Design review of the part built by this model. Coordinates are the model's own, in mm. A direction names the side the tool comes from. Give positions to 0.01 mm unless a question says otherwise; leave off trailing zeros. Loops run counter-clockwise (first coordinate to the right, second up) from the corner with the lowest first, then second, coordinate; pieces in that order, holes last. Notation, with made-up numbers: M -35.5,1 L -0.5,1 A20 ccw -0.5,25 Z; hole C -23.5,28.5 d8. An arc over 180 degrees is marked long. Use one line per item in the form item = value. Start each with the question number.
Autodesk Inventor part; units mm, degrees
ref_plane "YZ Plane" through (0, 0, 0) normal (1, 0, 0) x (0, 1, 0)
ref_plane "XZ Plane" through (0, 0, 0) normal (0, 1, 0) x (-1, 0, 0)
ref_plane "XY Plane" through (0, 0, 0) normal (0, 0, 1) x (1, 0, 0)
sketch "Sketch1" plane through (0, 0, 0) normal (0, 1, 0) x (-1, 0, 0)
  line L0 (25, 25) -> (-25, 25)
  line L1 (-25, 25) -> (-25, -25)
  line L2 (-25, -25) -> (25, -25)
  line L3 (25, -25) -> (25, 25)
  point P0 (0, 0)
  dimension "d0" = 50
  dimension "d1" = 50
  dimension "d2" = 25
  dimension "d3" = 25
extrude "Extrusion1" add sketch "Sketch1" along normal blind 7.5
sketch "Sketch2" plane through (0, 7.5, 0) normal (0, 1, 0) x (1, 0, 0)
  line L0 (-25, 25) -> (-25, -25)
  line L1 (25, -25) -> (25, 25)
  line L2 (-25, -25) -> (25, -25)
  line L3 (25, -25) -> (25, -17.5)
  line L4 (25, -17.5) -> (-25, -17.5)
  line L5 (-25, -17.5) -> (-25, -25)
  line L6 (-25, 25) -> (25, 25)
  line L7 (25, 25) -> (25, 17.5)
  line L8 (25, 17.5) -> (-25, 17.5)
  line L9 (-25, 17.5) -> (-25, 25)
  point P0 (0, 0)
  point P1 (-25, -17.5)
  point P2 (-25, 17.5)
  dimension "d6" = 7.5
  dimension "d7" = 7.5
  dimension "d8" = 25
extrude "Extrusion2" add sketch "Sketch2" along normal blind 120 contours L6 L1 L8 L0 | L4 L1 L2 L0
sketch "Sketch3" plane through (-25, 0, 25) normal (0, 0, 1) x (1, 0, 0)
  circle A0 centre (33, 97.5) radius 1.1
  circle A1 centre (33, 42) radius 1.1
  circle A2 centre (17, 42) radius 1.1
  circle A3 centre (17, 97.5) radius 1.1
  line L0 (50, 0) -> (50, 127.5)
  line L1 (0, 0) -> (0, 127.5)
  line L2 (0, 127.5) -> (50, 127.5)
  point P0 (25, 0)
  dimension "d11" = 2.2
  dimension "d12" = 2.2
  dimension "d13" = 2.2
  dimension "d14" = 2.2
  dimension "d15" = 55.5
  dimension "d17" = 55.5
  dimension "d18" = 17
  dimension "d19" = 17
  dimension "d20" = 17
  dimension "d21" = 17
  dimension "d22" = 30
  dimension "d23" = 30
extrude "Extrusion3" cut sketch "Sketch3" against normal through all
sketch "Sketch4" plane through (-25, 0, 25) normal (0, 0, 1) x (1, 0, 0)
  circle A0 centre (17, 97.5) radius 1.1
  circle A1 centre (17, 97.5) radius 3
  circle A2 centre (33, 97.5) radius 1.1
  circle A3 centre (33, 97.5) radius 3
  circle A4 centre (17, 42) radius 1.1
  circle A5 centre (17, 42) radius 3
  circle A6 centre (33, 42) radius 1.1
  circle A7 centre (33, 42) radius 3
  point P0 (25, 0)
  dimension "d26" = 6
  dimension "d27" = 6
  dimension "d28" = 6
  dimension "d29" = 6
extrude "Extrusion4" cut sketch "Sketch4" against normal blind 2.5 contours A1 | A2 | A3 | A5 | A7
sketch "Sketch5" plane through (0, 127.5, 0) normal (0, 1, 0) x (1, 0, 0)
  circle A0 centre (-20, -12.5) radius 1.6
  circle A1 centre (-20, 12.5) radius 1.6
  line L0 (-25, 17.5) -> (-25, -17.5)
  line L1 (-25, 17.5) -> (25, 17.5)
  line L2 (25, -17.5) -> (-25, -17.5)
  circle A2 centre (-20, -12.5) radius 5
  circle A3 centre (-20, 12.5) radius 5
  line L3 (-25, 17.5) -> (-25, 7.5)
  line L4 (-25, 7.5) -> (-20, 7.5)
  line L5 (25, 17.5) -> (-25, 17.5)
  line L6 (-7.9289, 17.5) -> (-16.4645, 8.9645)
  line L7 (-7.9289, 17.5) -> (9.8712, 17.5) construction
  line L8 (-25, 25) -> (-25, 17.5)
  line L9 (-25, 17.5) -> (-7.9289, 17.5)
  line L10 (-25, -17.5) -> (-25, -25)
  line L11 (-25, -17.5) -> (-25, -7.5)
  line L12 (-25, 25) -> (-25, -25)
  line L13 (-25, -7.5) -> (-20, -7.5)
  line L14 (-7.9289, -17.5) -> (-16.4645, -8.9645)
  line L15 (-7.9289, -17.5) -> (7.3912, -17.5) construction
  line L16 (-7.9289, -17.5) -> (-25, -17.5)
  point P0 (0, 0)
  dimension "d32" = 3.2
  dimension "d33" = 3.2
  dimension "d34" = 5
  dimension "d35" = 5
  dimension "d36" = 5
  dimension "d37" = 5
  dimension "d38" = 10
  dimension "d39" = 10
  dimension "d40" = 10
  dimension "d41" = 135
  dimension "d42" = 10
  dimension "d43" = 5
  dimension "d44" = 135
extrude "Extrusion5" add sketch "Sketch5" against normal blind 7.5
mirror "Mirror1" about plane through (0, 0, 0) normal (1, 0, 0) of "Extrusion5"
sketch "Sketch6" plane through (0, 0, 0) normal (0, -1, 0) x (1, 0, 0)
  circle A0 centre (-10, 0) radius 4.5
  circle A1 centre (10, 0) radius 4.5
  line L0 (0, 35) -> (0, -35)
  line L1 (25, 25) -> (25, -25)
  circle A2 centre (0, 0) radius 1
  point P0 (25, 0)
  dimension "Festo_Clips" = 9
  dimension "d48" = 9
  dimension "d49" = 0
  dimension "d50" = 10
  dimension "d51" = 10
  dimension "d52" = 0
  dimension "d77" = 2
extrude "Extrusion6" cut sketch "Sketch6" against normal blind 7.5
sketch "Sketch7" plane through (-25, 0, -25) normal (-1, 0, 0) x (0, 0, 1)
  circle A0 centre (3.75, 3.75) radius 1.5
  circle A1 centre (3.75, 63.75) radius 1.5
  circle A2 centre (3.75, 123.75) radius 1.5
  line L0 (0, 0) -> (0, 127.5)
  line L1 (0, 127.5) -> (17.5, 127.5)
  line L2 (0, 0) -> (50, 0)
  point P0 (25, 0)
  dimension "d55" = 3
  dimension "d56" = 3
  dimension "d57" = 3
  dimension "d58" = 3.75
  dimension "d59" = 3.75
  dimension "d60" = 3.75
  dimension "d61" = 3.75
  dimension "d62" = 3.75
  dimension "d63" = 63.75
extrude "Extrusion7" cut sketch "Sketch7" against normal blind 4
mirror "Mirror2" about plane through (0, 0, 0) normal (1, 0, 0) of "Extrusion7"
mirror "Mirror3" about plane through (0, 0, 0) normal (0, 0, 1) of "Extrusion7", "Mirror2"
sketch "Sketch8" plane through (25, 0, 25) normal (1, 0, 0) x (0, 0, -1)
  circle A0 centre (46.25, 3.75) radius 1.5
  circle A1 centre (46.25, 3.75) radius 2.5
  circle A2 centre (3.75, 3.75) radius 1.5
  circle A3 centre (3.75, 3.75) radius 2.5
  circle A4 centre (3.75, 63.75) radius 1.5
  circle A5 centre (3.75, 63.75) radius 2.5
  circle A6 centre (46.25, 63.75) radius 1.5
  circle A7 centre (46.25, 63.75) radius 2.5
  circle A8 centre (46.25, 123.75) radius 1.5
  circle A9 centre (46.25, 123.75) radius 2.5
  circle A10 centre (3.75, 123.75) radius 1.5
  circle A11 centre (3.75, 123.75) radius 2.5
  point P0 (25, 0)
  dimension "d66" = 5
  dimension "d67" = 5
  dimension "d68" = 5
  dimension "d69" = 5
  dimension "d70" = 5
  dimension "d71" = 5
extrude "Extrusion8" cut sketch "Sketch8" against normal blind 5.1 contours A0 | A1 | A2 | A3 | A4 | A5 | A6 | A7 | A8 | A9 | A10 | A11
mirror "Mirror4" about plane through (0, 0, 0) normal (1, 0, 0) of "Extrusion8"
chamfer "Chamfer1" distance 2 angle 45 8 edges at (0, 0, 25) (0, 0, -25) (0, 7.5, -17.5) (0, 7.5, 17.5) (16.4645, 120, -17.5) (16.4645, 120, 17.5) (-16.4645, 120, -17.5) (-16.4645, 120, 17.5)
mirror "Mirror5" about plane through (0, 0, 0) normal (0, 0, 1) of "Extrusion4"
equation "\"d6\" = Thickness"
equation "\"d7\" = Thickness"
equation "\"d45\" = Thickness"
equation "\"d48\" = Festo_Clips"
equation "\"d53\" = Thickness"
equation "\"d58\" = 0.5 * Thickness"
equation "\"d59\" = 0.5 * Thickness"
equation "\"d60\" = 0.5 * Thickness"
equation "\"d61\" = 0.5 * Thickness"
equation "\"d62\" = 0.5 * Thickness"
properties part number "Main_Cover"
Q1. Take a section at B-B on z = 12.5. Give the boundary of the cut face in (x, y).
Q2. The part is to be moulded in two halves that separate along Z. For faces 1 (the cylindrical face through (-7.41, 98.43, 20.04)), 2 (the cylindrical face through (18.11, 123.8, 7.87)), 3 (the flat face through (0, 64, 25)), say which applies: pulls with the +Z half, pulls with the -Z half, needs draft (parallel to the pull), parting line crosses it, or undercut.
Q3. Clearance check with flat-ended pins moving along their axes: pin 1 Ø2.5 at (x, y) = (-8, 42) entering from -Z; pin 2 Ø3.5 at (x, y) = (-8, 97.5) entering from +Z; pin 3 Ø1.5 at (y, z) = (3.5, 22.5) entering from -X. State where each tip first meets the part, or that it passes through.
Q4. Take a section at A-A on y = 72.5. Give the boundary of the cut face in (x, z).
Q5. For faces 4 (the cylindrical face through (22.486, 3.86, 23.748)), 5 (the flat face through (-12.14, 123.87, 13.29)), 6 (the cylindrical face through (-22.486, 3.64, -18.752)), 7 (the flat face through (-23, 124, -7.5)), list the 3-axis set-ups (+Z, -Z, +X, -X, +Y, -Y) from which the entire face can be reached by the end or side of a thin tool; tool diameter is ignored.
Q6. Wall thickness on probe 1 along Y at (x, z) = (-8, -19); probe 2 along Z at (x, y) = (-20, 124); probe 3 along Z at (x, y) = (11, 56.5): over which ranges is each line inside the solid? List them lowest first.
Response values:
q1.outline = M -25,0 L 25,0 L 25,7.5 L -25,7.5 Z; M -25,120 L -21.6,120 L -21.6,127.5 L -25,127.5 Z; M -18.4,120 L -12.93,120 L -12.93,127.5 L -18.4,127.5 Z; M 12.93,120 L 18.4,120 L 18.4,127.5 L 12.93,127.5 Z; M 21.6,120 L 25,120 L 25,127.5 L 21.6,127.5 Z
q2.face_1 = needs draft
q2.face_2 = undercut
q2.face_3 = pulls with the +Z half
q3.pin_1 = -22.5
q3.pin_2 = 22.5
q3.pin_3 = -19.9
q4.outline = M -25,-25 L 25,-25 L 25,-17.5 L -25,-17.5 Z; M -25,17.5 L 25,17.5 L 25,25 L -25,25 Z
q5.face_4 = +X
q5.face_5 = +Y
q5.face_6 = -X
q5.face_7 = +X, -X, +Y
q6.probe_1 = 0 to 40.9, 43.1 to 96.4, 98.6 to 127.5
q6.probe_2 = -25 to -23.74, -18.76 to -14.1, -10.9 to -7.5, 7.5 to 10.9, 14.1 to 18.76, 23.74 to 25
q6.probe_3 = -25 to -17.5, 17.5 to 25
